from build123d import *
from build123d import SkipClean  # not in build123d's __all__

# Parameters (mm, degrees)
F1_DEPTH = 7.62
F2_R     = 12.7
F2_R_2   = 9.398
F3_DEPTH = 38.1
F4_R     = 10.668
F4_R_2   = 9.398
F5_DEPTH = 12.7
F6_R     = 6.35
F7_DEPTH = 25.4
F8_SIZE2 = 1.3198227154
F8_SIZE  = 0.762
F9_R     = 0.762


# Not quite as in the source:
# - after a boolean that leaves OpenCascade's solid faulty, fix() repairs it


with BuildPart() as f1:
    # F0 (on Front) → F1 (new body)
    with BuildSketch(Plane.XZ):
        with BuildLine():
            ThreePointArc((-21.1420084076, -2.54), (-20.3980596318, -0.7439487758), (-18.6020084076, 0))
            Line((-18.6020084076, 0), (32.7059915924, 0))
            ThreePointArc((32.7059915924, 0), (35.4000684287, -1.1159231637), (36.5159915924, -3.81))
            Line((36.5159915924, -3.81), (36.5159915924, -8.89))
            Line((36.5159915924, -8.89), (34.3569915924, -8.89))
            Line((34.3569915924, -8.89), (34.3569915924, -4.318))
            ThreePointArc((34.3569915924, -4.318), (33.6874376942, -2.7015538982), (32.0709915924, -2.032))
            Line((32.0709915924, -2.032), (29.2769915924, -2.032))
            Line((29.2769915924, -2.032), (17.8469915924, -2.032))
            Line((17.8469915924, -2.032), (17.8469915924, -9.652))
            Line((17.8469915924, -9.652), (24.7049915924, -9.652))
            ThreePointArc((24.7049915924, -9.652), (27.937883796, -10.9911077964), (29.2769915924, -14.224))
            Line((29.2769915924, -14.224), (29.2769915924, -15.24))
            ThreePointArc((29.2769915924, -15.24), (29.6489659803, -16.1380256121), (30.5469915924, -16.51))
            Line((30.5469915924, -16.51), (42.8659915924, -16.51))
            ThreePointArc((42.8659915924, -16.51), (43.7640172045, -16.1380256121), (44.1359915924, -15.24))
            Line((44.1359915924, -15.24), (44.1359915924, 0))
            Line((44.1359915924, 0), (12.7, 127))
            ThreePointArc((12.7, 127), (0, 139.7), (-12.7, 127))
            Line((-12.7, 127), (-31.3020084076, 0))
            Line((-31.3020084076, 0), (-31.3020084076, -16.51))
            ThreePointArc((-31.3020084076, -16.51), (-30.9300340197, -17.4080256121), (-30.0320084076, -17.78))
            Line((-30.0320084076, -17.78), (-22.4120084076, -17.78))
            ThreePointArc((-22.4120084076, -17.78), (-21.5139827955, -17.4080256121), (-21.1420084076, -16.51))
            Line((-21.1420084076, -16.51), (-21.1420084076, -2.54))
        make_face()
        Polygon((13.8583155349, 10.2559253573), (-17.4904800951, 10.2559253573), (-17.9861974368, 10.2559253573), (-16.4103638381, 24.8740110546), align=None, mode=Mode.SUBTRACT)
        Polygon((30.8991490559, 10.2559253573), (-15.5502194539, 32.8530669212), (18.8005114427, 63.1991239488), align=None, mode=Mode.SUBTRACT)
        Polygon((16.8689347681, 72.4665825348), (-14.2382610105, 45.0233372929), (-10.1512422372, 82.9362176403), align=None, mode=Mode.SUBTRACT)
        Polygon((-7.1419274588, 110.8518689871), (8.8684540242, 110.8518689871), (14.6986516415, 82.8793242388), (-9.1010310551, 92.6784119132), align=None, mode=Mode.SUBTRACT)
    extrude(amount=F1_DEPTH)

    # F2 (on face) → F3 (join)
    with BuildSketch(Plane.XZ.offset(7.62)):
        with Locations((0, 127)):
            Circle(F2_R)
        with Locations((0, 127)):
            Circle(F2_R_2, mode=Mode.SUBTRACT)
    extrude(amount=-F3_DEPTH)

    # F4 (on face) → F5 (join)
    with BuildSketch(Plane(origin=(0, 30.48, 0), x_dir=(-1, 0, 0), z_dir=(0, 1, 0))):
        with Locations((0, 127)):
            Circle(F4_R)
        with Locations((0, 127)):
            Circle(F4_R_2, mode=Mode.SUBTRACT)
    with SkipClean():  # cleaning this boolean's faces spoils the solid; the shape is the same uncleaned
        extrude(amount=F5_DEPTH)

    # F6 (on face) → F7 (cut)
    with BuildSketch(Plane.XZ.offset(7.62)):
        with Locations((0, 127)):
            Circle(F6_R)
    extrude(amount=-F7_DEPTH, mode=Mode.SUBTRACT)

    add(f1.part.fix(), mode=Mode.REPLACE)

    # F8
    f8_edges = [f1.edges().sort_by_distance(p)[0] for p in [
        (-22.001004, -7.62, 63.5),
        (-31.302008, -7.62, -8.255),
        (-30.930034, -7.62, -17.408026),
        (-26.222008, -7.62, -17.78),
        (-21.513983, -7.62, -17.408026),
        (-21.142008, -7.62, -9.525),
        (-20.39806, -7.62, -0.743949),
        (7.051992, -7.62, 0),
        (35.400068, -7.62, -1.115923),
        (36.515992, -7.62, -6.35),
        (35.436492, -7.62, -8.89),
        (34.356992, -7.62, -6.604),
        (33.687438, -7.62, -2.701554),
        (24.958992, -7.62, -2.032),
        (17.846992, -7.62, -5.842),
        (21.275992, -7.62, -9.652),
        (27.937884, -7.62, -10.991108),
        (29.276992, -7.62, -14.732),
        (29.648966, -7.62, -16.138026),
        (36.706492, -7.62, -16.51),
        (43.764017, -7.62, -16.138026),
        (44.135992, -7.62, -7.62),
        (28.417996, -7.62, 63.5),
        (0, -7.62, 139.7),
        (-17.198281, -7.62, 17.564968),
        (-1.276024, -7.62, 17.564968),
        (-2.063941, -7.62, 10.255925),
        (1.315337, -7.62, 58.74496),
        (-12.194752, -7.62, 63.979777),
        (3.358846, -7.62, 77.7014),
        (24.84983, -7.62, 36.727525),
        (7.674465, -7.62, 21.554496),
        (1.625146, -7.62, 48.026095),
        (0.863263, -7.62, 110.851869),
        (11.783553, -7.62, 96.865597),
        (2.79881, -7.62, 87.778868),
        (-8.121479, -7.62, 101.76514),
        (-6.35, -7.62, 127),
    ]]
    f8_side = f1.faces().sort_by_distance((-20.273277, -7.62, 63.246935))[0]
    chamfer(f8_edges, length=F8_SIZE, length2=F8_SIZE2, reference=f8_side)

    # F9
    f9_edges = [f1.edges().sort_by_distance(p)[0] for p in [
        (10.668, 43.18, 127),
    ]]
    fillet(f9_edges, radius=F9_R)


solid = f1.part
Build history of the part. All positions in model axes, mm. A direction names the side the tool comes from. Round coordinates to 2 decimals unless told otherwise and drop trailing zeros. Order: outer loops, then holes, each group sorted by start corner. A loop starts at its lowest first (then second) coordinate and runs counter-clockwise, first axis right, second up. Notation, with made-up numbers: M 9.5,76.5 L 26.5,76.5 A14 cw 26.5,86.5 Z; hole C 25.25,-30 d1. An arc over 180 degrees is marked long. Use CSV: the item, a comma, the result in double quotes. Start each with the question number.
(1) Mould opens along X. For faces 1 (the face through (37, -3, -16.51)), 2 (the face through (44.136, -3, -8)), 3 (the face through (36.516, -3, -6)) say: +X half, -X half, draft (parallel to the pull), parting line (faces both ways), or undercut.
(2) Cut at C-C on x = 0. State how many separate pieces and enclosed holes the cut face has, then the cut area to 3 significant figures.
(3) Cut at A-A on z = 20. List the corners of the cut face in (x, y).
(4) Drill centre lines: probe 1 along X at (y, z) = (15, 127); probe 2 along Z at (x, y) = (0, -3); probe 3 along Z at (x, y) = (-0.5, 10). Where is each one in solid material? Low to high.
(5) Tool access for faces 4 (the face through (27.902, -3.106, -10.956)), 5 (the face through (-20.626, -6.804, -0.56)), 6 (the face through (-7, 30.48, 136)), 7 (the face through (-17.21, -3.11, 17.46)), 8 (the face through (-12.65, -6.95, 63.25)): list every direction of +Z, -Z, +X, -X, +Y, -Y with a clear straight run to the whole face (end or side of a thin tool).
(6) Cut at B-B on y = 24. List the corners of the cut face in (x, z), then the cut area to 3 significant figures.
(7) Flat gauge pins, fed straight in: P1, Ø1.5, axis at x = 5, y = 0.5, coming from the +Z side; P2, Ø7.5, axis at x = 3, z = 130.5, coming from the +Y side; P3, Ø7, axis at x = -3.5, y = -1.5, coming from the +Z side; P4, Ø10, axis at y = 4.5, z = 98, coming from the -X side. Where does each tip first touch, or does it go through?
Findings:
1,face 1,"draft"
1,face 2,"+X half"
1,face 3,"undercut"
2,separate pieces,"6"
2,enclosed holes,"0"
2,area,"651 mm^2"
3,outline,"M -28.37,-6.3 L -27.6,-7.62 L -17.7,-7.62 L -16.94,-6.3 L -16.94,0 L -28.37,0 Z; M -6.32,-6.3 L -4.57,-7.62 L 9.13,-7.62 L 10.87,-6.3 L 10.87,0 L -6.32,0 Z; M 28.67,-6.3 L 29.45,-7.62 L 38.4,-7.62 L 39.19,-6.3 L 39.19,0 L 28.67,0 Z"
4,probe 1,"x = -12.7 to -9.4, 9.4 to 12.7"
4,probe 2,"z = 0 to 10.26, 16.95 to 25.29, 46.59 to 57.58, 79 to 88.93, 110.85 to 120.65, 133.35 to 139.7"
4,probe 3,"z = 114.31 to 117.62, 136.38 to 139.69"
5,face 4,"-Z, +Y, -Y"
5,face 5,"-Z, -Y"
5,face 6,"+Y"
5,face 7,"+Y, -Y"
5,face 8,"-Y"
6,outline,"C 0,127 d25.4; hole C 0,127 d18.8"
6,area,"229 mm^2"
7,P1,"stops at z = 138.97"
7,P2,"stops at y = 0"
7,P3,"stops at z = 139.7"
7,P4,"stops at x = -17.27"
